Input: part model. Units: mm. Frame: model coordinates. Face numbers are marked on the shaded views. A direction names the side the tool comes from. Give positions to 0.01 mm unless a question says otherwise; leave off trailing zeros. Write each loop counter-clockwise with the first axis right and the second up, starting at its lowest first coordinate (ties: lowest second). Pieces come first, ordered by that corner, then holes. Notation, with made-up numbers: (67.5, 61.25) -> (103.5, 61.25) arc R22 ccw to (103.5, 97.25) -> close; hole circle Ø7 at (7.25, 4). An arc over 180 degrees is marked (long way). Answer as a JSON object with one key per item and string values. Group by question number.
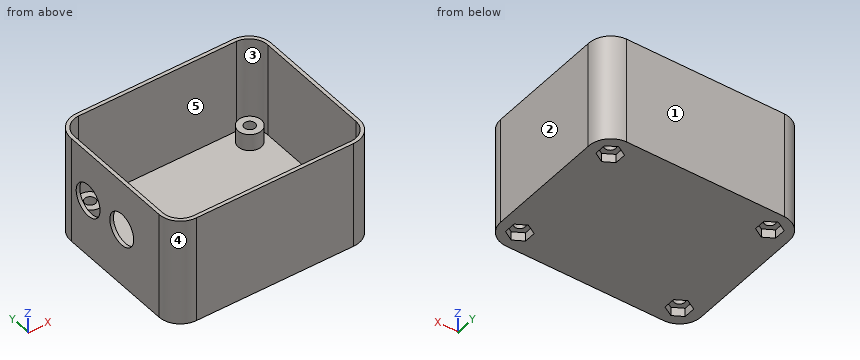
from build123d import *

# Parameters (mm, degrees)
SKETCH1_R           = 1.5
BOSS_EXTRUDE2_DEPTH = 3.75
BOSS_EXTRUDE3_DEPTH = 30
CUT_EXTRUDE1_DEPTH  = 2.4
SKETCH3_R           = 3.25
SKETCH3_R_2         = 1.5
BOSS_EXTRUDE4_DEPTH = 4.65
SKETCH4_R           = 4.5
CUT_EXTRUDE2_DEPTH  = 1


with BuildPart() as part:
    # Sketch1 → Boss-Extrude2 (new body)
    # profile 1 of 2: a face of its own
    with BuildSketch(Plane.XY):
        with BuildLine():
            Line((55.205, 35.540044664), (55.205, 2.5))
            ThreePointArc((55.205, 2.5), (53.740533906, -1.035533906), (50.205, -2.5))
            Line((50.205, -2.5), (6.31, -2.5))
            ThreePointArc((6.31, -2.5), (2.774466094, -1.035533906), (1.31, 2.5))
            Line((1.31, 2.5), (1.31, 35.540044664))
            ThreePointArc((1.31, 35.540044664), (2.66894591, 39.245525041), (6.250024717, 40.9048))
            Line((6.250024717, 40.9048), (50.264975283, 40.9048))
            ThreePointArc((50.264975283, 40.9048), (53.84605409, 39.245525041), (55.205, 35.540044664))
        make_face()
        with BuildLine():
            ThreePointArc((3.81, 2.5), (4.542233047, 0.732233047), (6.31, 0))
            Line((6.31, 0), (50.205, 0))
            ThreePointArc((50.205, 0), (51.972766953, 0.732233047), (52.705, 2.5))
            Line((52.705, 2.5), (52.705, 35.6))
            ThreePointArc((52.705, 35.6), (52.03588526, 37.520159965), (50.205, 38.4048))
            Line((50.205, 38.4048), (6.31, 38.4048))
            ThreePointArc((6.31, 38.4048), (4.47911474, 37.520159965), (3.81, 35.6))
            Line((3.81, 35.6), (3.81, 2.5))
        make_face(mode=Mode.SUBTRACT)
    # profile 2 of 2: a face of its own
    with BuildSketch(Plane.XY):
        with BuildLine():
            Line((3.81, 35.6), (3.81, 2.5))
            ThreePointArc((3.81, 2.5), (4.542233047, 0.732233047), (6.31, 0))
            Line((6.31, 0), (50.205, 0))
            ThreePointArc((50.205, 0), (51.972766953, 0.732233047), (52.705, 2.5))
            Line((52.705, 2.5), (52.705, 35.6))
            ThreePointArc((52.705, 35.6), (52.03588526, 37.520159965), (50.205, 38.4048))
            Line((50.205, 38.4048), (6.31, 38.4048))
            ThreePointArc((6.31, 38.4048), (4.47911474, 37.520159965), (3.81, 35.6))
        make_face()
        with Locations((6.096, 36.2712)):
            Circle(SKETCH1_R, mode=Mode.SUBTRACT)
        with Locations((50.5968, 36.2712)):
            Circle(SKETCH1_R, mode=Mode.SUBTRACT)
        with Locations((50.5968, 2.1336)):
            Circle(SKETCH1_R, mode=Mode.SUBTRACT)
        with Locations((6.096, 2.1336)):
            Circle(SKETCH1_R, mode=Mode.SUBTRACT)
    extrude(amount=BOSS_EXTRUDE2_DEPTH)

    # Sketch1<3> → Boss-Extrude3 (add)
    with BuildSketch(Plane.XY):
        with BuildLine():
            Line((56.205, 35.52036079), (56.205, 2.5))
            ThreePointArc((56.205, 2.5), (54.447640687, -1.742640687), (50.205, -3.5))
            Line((50.205, -3.5), (6.31, -3.5))
            ThreePointArc((6.31, -3.5), (2.067359313, -1.742640687), (0.31, 2.5))
            Line((0.31, 2.5), (0.31, 35.52036079))
            ThreePointArc((0.31, 35.52036079), (1.947918213, 39.938710907), (6.230334295, 41.9048))
            Line((6.230334295, 41.9048), (50.284665705, 41.9048))
            ThreePointArc((50.284665705, 41.9048), (54.567081787, 39.938710907), (56.205, 35.52036079))
        make_face()
        with BuildLine():
            ThreePointArc((55.205, 35.540044664), (53.84605409, 39.245525041), (50.264975283, 40.9048))
            Line((50.264975283, 40.9048), (6.250024717, 40.9048))
            ThreePointArc((6.250024717, 40.9048), (2.66894591, 39.245525041), (1.31, 35.540044664))
            Line((1.31, 35.540044664), (1.31, 2.5))
            ThreePointArc((1.31, 2.5), (2.774466094, -1.035533906), (6.31, -2.5))
            Line((6.31, -2.5), (50.205, -2.5))
            ThreePointArc((50.205, -2.5), (53.740533906, -1.035533906), (55.205, 2.5))
            Line((55.205, 2.5), (55.205, 35.540044664))
        make_face(mode=Mode.SUBTRACT)
    extrude(amount=BOSS_EXTRUDE3_DEPTH)

    # Sketch2 → Cut-Extrude1 (cut)
    with BuildSketch(Plane(origin=(0, 0, 0), x_dir=(-1, 0, 0), z_dir=(0, 0, -1))):
        Polygon((-50.5968, 5.366761507), (-53.3968, 3.750180754), (-53.3968, 0.517019246), (-50.5968, -1.099561507), (-47.7968, 0.517019246), (-47.7968, 3.750180754), align=None)
        Polygon((-47.7968, 37.887780754), (-50.5968, 39.504361507), (-53.3968, 37.887780754), (-53.3968, 34.654619246), (-50.5968, 33.038038493), (-47.7968, 34.654619246), align=None)
        Polygon((-6.096, 39.504361507), (-8.896, 37.887780754), (-8.896, 34.654619246), (-6.096, 33.038038493), (-3.296, 34.654619246), (-3.296, 37.887780754), align=None)
        Polygon((-6.096, 5.366761507), (-8.896, 3.750180754), (-8.896, 0.517019246), (-6.096, -1.099561507), (-3.296, 0.517019246), (-3.296, 3.750180754), align=None)
    extrude(amount=-CUT_EXTRUDE1_DEPTH, mode=Mode.SUBTRACT)

    # Sketch3 → Boss-Extrude4 (add)
    # profile 1 of 4: a face of its own
    with BuildSketch(Plane.XY.offset(3.75)):
        with Locations((6.096, 36.2712)):
            Circle(SKETCH3_R)
        with Locations(Location((6.096, 36.2712, 0), (0, 0, 180))):
            Circle(SKETCH3_R_2, mode=Mode.SUBTRACT)
    # profile 2 of 4: a face of its own
    with BuildSketch(Plane.XY.offset(3.75)):
        with Locations((6.096, 2.1336)):
            Circle(SKETCH3_R)
        with Locations(Location((6.096, 2.1336, 0), (0, 0, 180))):
            Circle(SKETCH3_R_2, mode=Mode.SUBTRACT)
    # profile 3 of 4: a face of its own
    with BuildSketch(Plane.XY.offset(3.75)):
        with Locations((50.5968, 2.1336)):
            Circle(SKETCH3_R)
        with Locations(Location((50.5968, 2.1336, 0), (0, 0, 180))):
            Circle(SKETCH3_R_2, mode=Mode.SUBTRACT)
    # profile 4 of 4: a face of its own
    with BuildSketch(Plane.XY.offset(3.75)):
        with Locations((50.5968, 36.2712)):
            Circle(SKETCH3_R)
        with Locations(Location((50.5968, 36.2712, 0), (0, 0, 180))):
            Circle(SKETCH3_R_2, mode=Mode.SUBTRACT)
    extrude(amount=BOSS_EXTRUDE4_DEPTH)

    # Sketch4 → Cut-Extrude2 (cut)
    with BuildSketch(Plane.ZY.offset(-0.31)):
        with Locations(Location((16.15, 29.21, 0), (0, 0, 270))):
            Circle(SKETCH4_R)
        with Locations(Location((16.15, 16.51, 0), (0, 0, 270))):
            Circle(SKETCH4_R)
    extrude(amount=-CUT_EXTRUDE2_DEPTH, mode=Mode.SUBTRACT)


solid = part.part
1. Section A-A (y = 16.51). Return the cut outline in (x, z) (3 decimals).
2. Section C-C (z = 16.15). Return the cut outline in (x, y) (3 decimals).
3. Contact query for flat-ended pins moving along their axis: pin 1 Ø2 at (x, y) = (5.5, 0.5) entering from +Z; pin 2 Ø10 at (y, z) = (10.5, 18.5) entering from +X (3 decimals); pin 3 Ø5 at (x, y) = (6.1, 2.13) entering from -Z. Output: stop coordinate, or through.
4. Reachability of the marked faces 4 and 5 from +Z, -Z, +X, -X, +Y, -Y: full face, straight path, thin tool, end or side. Return the list, or none.
5. Section B-B (z = 22.75). Return the cut outline in (x, y) (3 decimals), plus the area to 3 significant figures.
6. Section D-D (y = 23.5). Return the cut outline in (x, z) (3 decimals), plus the area to 3 significant figures.
7. Line query: line 1 (Y direction, x = 9, z = 12); line 2 (X direction, y = 20.5, z = 8.75) (3 decimals); line 3 (Y direction, x = 53, z = 6.5). Output: solid intervals per line, ascending.
8. Mould query, pull axis X, two halves, no side actions, for the marked faces 1, 2 and 3. Classes: pulls with the +X half, pulls with the -X half, needs draft (parallel to the pull), parting line crosses it, or undercut.
Working result:
{
 "1": {"outline": "(0.31, 0) -> (56.205, 0) -> (56.205, 30) -> (55.205, 30) -> (55.205, 3.75) -> (1.31, 3.75) -> (1.31, 11.65) -> (0.31, 11.65) -> close; (0.31, 20.65) -> (1.31, 20.65) -> (1.31, 30) -> (0.31, 30) -> close"},
 "2": {"outline": "(0.31, 2.5) arc R6 ccw to (6.31, -3.5) -> (50.205, -3.5) arc R6 ccw to (56.205, 2.5) -> (56.205, 35.52) arc R6.157 ccw to (50.285, 41.905) -> (6.23, 41.905) arc R6.157 ccw to (0.31, 35.52) -> (0.31, 33.71) -> (1.31, 33.71) -> (1.31, 35.54) arc R5.157 cw to (6.25, 40.905) -> (50.265, 40.905) arc R5.157 cw to (55.205, 35.54) -> (55.205, 2.5) arc R5 cw to (50.205, -2.5) -> (6.31, -2.5) arc R5 cw to (1.31, 2.5) -> (1.31, 12.01) -> (0.31, 12.01) -> close; (0.31, 21.01) -> (1.31, 21.01) -> (1.31, 24.71) -> (0.31, 24.71) -> close"},
 "3": {"pin 1": "stops at z = 8.4", "pin 2": "stops at x = 56.205", "pin 3": "stops at z = 2.4"},
 "4": {"face 4": "+Z, -Z, -X, -Y", "face 5": "+Z"},
 "5": {"outline": "(0.31, 2.5) arc R6 ccw to (6.31, -3.5) -> (50.205, -3.5) arc R6 ccw to (56.205, 2.5) -> (56.205, 35.52) arc R6.157 ccw to (50.285, 41.905) -> (6.23, 41.905) arc R6.157 ccw to (0.31, 35.52) -> close; hole (1.31, 2.5) arc R5 ccw to (6.31, -2.5) -> (50.205, -2.5) arc R5 ccw to (55.205, 2.5) -> (55.205, 35.54) arc R5.157 ccw to (50.265, 40.905) -> (6.25, 40.905) arc R5.157 ccw to (1.31, 35.54) -> close", "area": "189 mm^2"},
 "6": {"outline": "(0.31, 0) -> (56.205, 0) -> (56.205, 30) -> (55.205, 30) -> (55.205, 3.75) -> (1.31, 3.75) -> (1.31, 30) -> (0.31, 30) -> close", "area": "262 mm^2"},
 "7": {"line 1": "y = -3.5 to -2.5, 40.9 to 41.9", "line 2": "x = 0.31 to 1.31, 55.205 to 56.205", "line 3": "y = -2.81 to -1.65, -0.05 to 4.32, 34.08 to 38.46, 39.98 to 41.16"},
 "8": {"face 1": "needs draft", "face 2": "pulls with the +X half", "face 3": "undercut"}
}
